Geometry: final body of the model. Coordinates: model frame, mm. A direction names the side the tool comes from. Give positions to 0.01 mm unless a question says otherwise; leave off trailing zeros. Order: outer loops, then holes, each group sorted by start corner. A loop starts at its lowest first (then second) coordinate and runs counter-clockwise, first axis right, second up. Notation, with made-up numbers: M -16,-27 L 20,-27 A7 cw 20,-15 Z; hole C -21.75,67 d2. An arc over 180 degrees is marked long. One line per item, written item: value. Start each with the question number.
Autodesk Inventor part; units mm, degrees
ref_plane "YZ Plane" through (0, 0, 0) normal (1, 0, 0) x (0, 1, 0)
ref_plane "XZ Plane" through (0, 0, 0) normal (0, 1, 0) x (-1, 0, 0)
ref_plane "XY Plane" through (0, 0, 0) normal (0, 0, 1) x (1, 0, 0)
sketch "Sketch1" plane through (0, 0, 0) normal (0, 0, 1) x (1, 0, 0)
  circle A0 centre (0, 0) radius 24.5
  dimension "d0" = 49
extrude "Extrusion1" add sketch "Sketch1" along normal blind 110
sketch "Sketch2" plane through (0, 0, 110) normal (0, 0, 1) x (1, 0, 0)
  circle A0 centre (0, 0) radius 24.5
  circle A1 centre (0, 0) radius 14
  dimension "d3" = 28
extrude "Extrusion2" cut sketch "Sketch2" against normal blind 15
sketch "Sketch3" plane through (0, 0, 95) normal (0, 0, 1) x (1, 0, 0)
  circle A0 centre (0, 0) radius 24.5
  circle A1 centre (0, 0) radius 22
  dimension "d6" = 44
extrude "Extrusion3" cut sketch "Sketch3" against normal blind 60
sketch "Sketch4" plane through (0, 0, 0) normal (0, 0, -1) x (-1, 0, 0)
  circle A0 centre (0, 0) radius 24.5
  circle A1 centre (0, 0) radius 10
  dimension "d9" = 20
extrude "Extrusion4" cut sketch "Sketch4" against normal blind 17
chamfer "Chamfer1" distance 11 angle 45 1 edges at (-24.5, 0, 17) measured on face at (19.3325, 2.7521, 17)
sketch "Sketch5" plane through (0, 0, 95) normal (0, 0, 1) x (1, 0, 0)
  circle A0 centre (0, 0) radius 22
  circle A1 centre (0, 0) radius 14
extrude "Extrusion5" cut sketch "Sketch5" against normal blind 1
sketch "Sketch6" plane through (0, 0, 0) normal (0, 0, -1) x (-1, 0, 0)
  circle A0 centre (0, 0) radius 10
extrude "Extrusion6" cut sketch "Sketch6" against normal blind 1
sketch "Sketch7" plane through (0, 0, 1) normal (0, 0, -1) x (-1, 0, 0)
  circle A0 centre (0, 0) radius 10
  circle A1 centre (0, 0) radius 8
  dimension "d22" = 16
extrude "Extrusion7" cut sketch "Sketch7" against normal blind 16
sketch "Sketch8" plane through (0, 0, 35) normal (0, 0, 1) x (1, 0, 0)
  circle A0 centre (0, 0) radius 22
  circle A1 centre (0, 0) radius 24.5
extrude "Extrusion8" cut sketch "Sketch8" against normal blind 3
sketch "Sketch9" plane through (0, 0, 0) normal (0, 1, 0) x (-1, 0, 0)
  line L0 (22, 32) -> (-22, 32)
  line L1 (-22, 40) -> (-19, 40)
  line L2 (-19, 40) -> (-19, 32)
  line L3 (-19, 32) -> (-22, 32)
  line L4 (-22, 32) -> (-22, 40)
  line L5 (0, 0) -> (0, 69)
  point P0 (22, 69)
  point P1 (-22, 69)
  dimension "d27" = 8
  dimension "d28" = 38
  dimension "d29" = 3
revolve "Revolution1" cut sketch "Sketch9" angle 360 about axis through (0, 0, 0) along (0, 0, 1)
sketch "Sketch11" plane through (0, 0, 94) normal (0, 0, 1) x (1, 0, 0)
  circle A0 centre (0, 0) radius 22
  circle A1 centre (0, 0) radius 21
  dimension "d31" = 42
extrude "Extrusion9" cut sketch "Sketch11" against normal blind 30
chamfer "Chamfer3" distance 30 angle 6 1 edges at (-21, 0, 94) measured on face at (20.7281, -3.3686, 74)
sketch "Sketch12" plane through (0, 0, 64) normal (0, 0, 1) x (1, 0, 0)
  circle A0 centre (0, 0) radius 21
  circle A1 centre (0, 0) radius 22
extrude "Extrusion10" cut sketch "Sketch12" against normal blind 28
sketch "Sketch13" plane through (0, 0, 110) normal (0, 0, 1) x (1, 0, 0)
  circle A0 centre (0, 0) radius 14
hole "Hole1" at (0, 0, 110) direction (0, 0, -1) diameter 6.401 depth 35 tip angle 118 countersink diameter 10 countersink angle 60
sketch "Sketch14" plane through (0, 0, 1) normal (0, 0, -1) x (-1, 0, 0)
  circle A0 centre (0, 0) radius 8
hole "Hole2" at (0, 0, 1) direction (0, 0, 1) diameter 10 depth 32 tip angle 118 countersink diameter 11 countersink angle 60
sketch "Sketch16" plane through (0, 0, 110) normal (0, 0, 1) x (1, 0, 0)
  circle A0 centre (0, 0) radius 14
  circle A1 centre (0, 0) radius 10.5
  dimension "d56" = 21
extrude "Extrusion11" cut sketch "Sketch16" against normal blind 16
sketch "Sketch17" plane through (0, 0, 0) normal (1, 0, 0) x (0, 1, 0)
  line L0 (10.5, 94) -> (-10.5, 94)
  line L1 (10.5, 110) -> (-10.5, 110)
  line L2 (10.5, 94) -> (9.5, 94)
  line L3 (9.5, 94) -> (9.5, 100)
  line L4 (9.5, 100) -> (10.5, 100)
  line L5 (10.5, 100) -> (10.5, 94)
  line L6 (0, 110) -> (0, 0)
  dimension "d59" = 6
  dimension "d60" = 1
revolve "Revolution3" cut sketch "Sketch17" angle 360 about axis through (0, 0, 110) along (0, 0, -1)
thread "Thread1"
chamfer "Chamfer4" distance 1 angle 45 1 edges at (-10.5, 0, 110)
chamfer "Chamfer5" distance 0.5 angle 45 1 edges at (8, 0, 1)
fillet "Fillet1" radius 0.5 1 edges at (-17.8474, 0, 94)
sketch "Sketch18" plane through (0, 0, 0) normal (1, 0, 0) x (0, 1, 0)
  circle A0 centre (0, 9) radius 1.5
  line L0 (7.5, 1) -> (-7.5, 1)
  point P0 (0, 0)
  dimension "d71" = 3
  dimension "d72" = 8
extrude "Extrusion12" cut sketch "Sketch18" along normal mid plane 25
properties part number "EIXO DA BETONEIRA(21)" material "Carbon Steel"
Q1. Section query A-A on z = 80. Return loops of the section in (x, y).
Q2. Set-up query: faces 4 (the face through (10, 3.2, 104.6)), 5 (the face through (-16, -11, 40)), 6 (the face through (6.36, -1.5, 8.93)). Return all of +Z, -Z, +X, -X, +Y, -Y with unobstructed straight access to the full face (end or side cutting, diameter ignored); none if empty.
Q3. Mould query, pull axis Y, two halves, no side actions, for faces 1 (the face through (13.17, -20.66, 29.97)), 2 (the face through (-6, -6, 17)), 3 (the face through (-0.54, 0.12, 73.41)). Classes: +Y half, -Y half, draft (parallel to the pull), parting line (faces both ways), or undercut.
Q4. Ray query, line 1 along X through (y, z) = (0, 15); line 2 along Z through (x, y) = (-5.95, 0); line 3 along Y through (x, z) = (0, 90). Return the intervals inside material, ascending. Write a range as [from, to].
Q5. Contact query for flat-ended pins moving along their axis: pin 1 (5 mm diameter, centred on y = 0, z = 9, fed in from +X); pin 2 (8 mm diameter, centred on x = 0, y = -17, fed in from -Z); pin 3 (5 mm diameter, centred on x = -9.5, y = 17, fed in from +Z). Output: stop coordinate, or through.
Results below:
1. outline: C 0,0 d38.64; hole C 0,0 d6.4
2. face 4: +Z
2. face 5: none
2. face 6: +X, -X
3. face 1: parting line
3. face 2: draft
3. face 3: undercut
4. line 1: [-8, -5], [5, 8]
4. line 2: [1, 7.5], [10.5, 110]
4. line 3: [-18.27, -3.2], [3.2, 18.27]
5. pin 1: x = 8
5. pin 2: z = 17
5. pin 3: z = 94
